```python
from build123d import *

# Parameters (mm, degrees)
F_6_CLEARANCE_HOLE1_D     = 3.7973
F_6_CLEARANCE_HOLE1_DEPTH = 25.4
F_6_CLEARANCE_HOLE1_TIP   = 1.140824014


with BuildPart() as part:
    # Sketch2 → Revolve1 (revolve)
    with BuildSketch(Plane(origin=(0, 0, 0), x_dir=(0, 0, -1), z_dir=(1, 0, 0))):
        Polygon((0, 71.4375), (2.54, 69.85), (19.05, 69.85), (19.05, 72.9615), (6.35, 72.9615), (6.35, 76.2635), (19.05, 76.2635), (19.05, 79.375), (4.7625, 79.375), (4.7625, 88.9), (0, 88.9), align=None)
    revolve(axis=Axis((0, 0, 0), (0, 0, -1)))

    # #6 Clearance Hole1
    with Locations(Plane(origin=(0, 0, -4.7625), x_dir=(-1, 0, 0), z_dir=(0, 0, -1))):
        with Locations((0, -84.1375), (80.01951764, -25.999917364), (49.454781665, 68.068667364), (-80.01951764, -25.999917364), (-49.454781665, 68.068667364)):
            Hole(F_6_CLEARANCE_HOLE1_D / 2, depth=F_6_CLEARANCE_HOLE1_DEPTH)
            with Locations((0, 0, -(F_6_CLEARANCE_HOLE1_DEPTH + F_6_CLEARANCE_HOLE1_TIP / 2))):  # 118° drill point
                Cone(0, F_6_CLEARANCE_HOLE1_D / 2, F_6_CLEARANCE_HOLE1_TIP, mode=Mode.SUBTRACT)


solid = part.part
```
Source: CAD feature listing. Evaluate the final solid. Frame: model axes, mm. A direction names the side the tool comes from. Coordinates: 2 decimals unless noted, no trailing zeros. One line per item, written item: value. Start each with the question number.
Q1. Set-up query: faces 5 (the face through (-42.503, -55.431, -10.911)), 6 (the face through (60, 53, -4.762)). Return all of +Z, -Z, +X, -X, +Y, -Y with unobstructed straight access to the full face (end or side cutting, diameter ignored); none if empty.
Q2. Contact query for flat-ended pins moving along their axis: P1, Ø1.5, axis at x = 43, z = -4, coming from the +Y side; P2, Ø10, axis at y = -27, z = -2.5, coming from the -X side; P3, Ø4, axis at y = -9, z = -8, coming from the +X side. Output: stop coordinate, or through.
Q3. Line query: line 1 along X through (y, z) = (24, -13.75); line 2 along X through (y, z) = (-11, -12.5); line 3 along Y through (x, z) = (-40.5, -18). Output: solid intervals per line, ascending.
Q4. Mould query, pull axis Y, two halves, no side actions, for faces 1 (the face through (3.21, -72.89, -12.61)), 2 (the face through (23.84, 75.71, -11.81)), 3 (the face through (-78.21, -25.43, -2.35)), 4 (the face through (-72, 0, 0)). Classes: pulls with the +Y half, pulls with the -Y half, needs draft (parallel to the pull), parting line crosses it, or undercut.
Q5. Section query B-B, the plane z = -9. Give the number of separate pieces and of enclosed holes in the cut face, and give its area (3 significant figures).
Results:
1. face 5: +Z, -Z
1. face 6: -Z
2. P1: y = 78.22
2. P2: x = -86.13
2. P3: x = 79.07
3. line 1: -75.66 to -72.39, -68.9 to -65.6, 65.6 to 68.9, 72.39 to 75.66
3. line 2: -78.61 to -75.47, -72.13 to -68.98, 68.98 to 72.13, 75.47 to 78.61
3. line 3: -68.27 to -64.62, -60.69 to -56.91, 56.91 to 60.69, 64.62 to 68.27
4. face 1: undercut
4. face 2: parting line crosses it
4. face 3: undercut
4. face 4: needs draft
5. separate pieces: 2
5. enclosed holes: 2
5. area: 2,920 mm^2
